from build123d import *

# Parameters (mm, degrees)
EXTRUDE1_DEPTH          = 0.25
FILLET1_R               = 0.25
CUT_EXTRUDE1_DEPTH      = 31.234789562
CUT_EXTRUDE1_DEPTH_BACK = 31.234789562
SKETCH3_W               = 12
SKETCH3_H               = 2.8


with BuildPart() as part:
    # Sketch1 → Revolve1 (revolve)
    with BuildSketch(Plane(origin=(0, 0, 0), x_dir=(0, 0, -1), z_dir=(1, 0, 0)), mode=Mode.PRIVATE) as revolve1_sk:
        with BuildLine():
            Line((0, 1.45), (2.15, 1.45))
            Line((2.15, 1.45), (2.15, 1.599999975))
            Line((2.15, 1.599999975), (3.15, 1.599999975))
            Line((3.15, 1.599999975), (3.15, 0))
            Line((3.15, 0), (-1.45, 0))
            ThreePointArc((-1.45, 0), (-1.025304833, 1.025304833), (0, 1.45))
        make_face()
    revolve(revolve1_sk.sketch.rotate(Axis((0, 0, 0), (0, 0, -1)), 90), axis=Axis((0, 0, 0), (0, 0, -1)))

    # Sketch2 → Extrude1 (add, symmetric)
    with BuildSketch(Plane(origin=(0, 0, 0), x_dir=(0, 0, -1), z_dir=(1, 0, 0))):
        with BuildLine():
            Line((3.15, 1.026953873), (3.95, 1.4))
            Line((3.95, 1.4), (6.15, 1.4))
            Line((6.15, 1.4), (6.15, 1.5))
            Line((6.15, 1.5), (7.15, 1.5))
            Line((7.15, 1.5), (7.15, 1.4))
            Line((7.15, 1.4), (30.15, 1.4))
            Line((30.15, 1.4), (30.15, 0.9))
            Line((30.15, 0.9), (7.15, 0.9))
            Line((7.15, 0.9), (7.15, 0.8))
            Line((7.15, 0.8), (6.15, 0.8))
            Line((6.15, 0.8), (6.15, 0.9))
            Line((6.15, 0.9), (4.05, 0.9))
            ThreePointArc((4.05, 0.9), (3.979289322, 0.870710678), (3.95, 0.8))
            Line((3.95, 0.8), (3.95, 0.5))
            Line((3.95, 0.5), (3.15, 0.5))
            Line((3.15, 0.5), (3.15, 1.026953873))
        make_face()
        with BuildLine():
            Line((3.95, -0.8), (3.95, -0.5))
            Line((3.95, -0.5), (3.15, -0.5))
            Line((3.15, -0.5), (3.15, -1.026953873))
            Line((3.15, -1.026953873), (3.95, -1.4))
            Line((3.95, -1.4), (6.15, -1.4))
            Line((6.15, -1.4), (6.15, -1.5))
            Line((6.15, -1.5), (7.15, -1.5))
            Line((7.15, -1.5), (7.15, -1.4))
            Line((7.15, -1.4), (30.15, -1.4))
            Line((30.15, -1.4), (30.15, -0.9))
            Line((30.15, -0.9), (7.15, -0.9))
            Line((7.15, -0.9), (7.15, -0.8))
            Line((7.15, -0.8), (6.15, -0.8))
            Line((6.15, -0.8), (6.15, -0.9))
            Line((6.15, -0.9), (4.05, -0.9))
            ThreePointArc((4.05, -0.9), (3.979289322, -0.870710678), (3.95, -0.8))
        make_face()
    extrude(amount=EXTRUDE1_DEPTH, both=True)

    # Fillet1
    fillet1_edges = [part.edges().sort_by_distance(p)[0] for p in [
        (-0.25, 0.763476937, -3.15),
        (0, 1.026953873, -3.15),
        (0, 0.5, -3.15),
        (0.25, 0.763476937, -3.15),
        (-0.25, -0.763476937, -3.15),
        (0, -0.5, -3.15),
        (0, -1.026953873, -3.15),
        (0.25, -0.763476937, -3.15),
    ]]
    fillet(fillet1_edges, radius=FILLET1_R)

    # Sketch3 → Cut-Extrude1 (cut, two sides: drawn at the far end of the back side and taken through both)
    with BuildSketch(Plane(origin=(0, 0, 0), x_dir=(0, 0, -1), z_dir=(1, 0, 0)).offset(-CUT_EXTRUDE1_DEPTH_BACK)):
        with Locations((24.15, 0)):
            Rectangle(SKETCH3_W, SKETCH3_H)
    extrude(amount=CUT_EXTRUDE1_DEPTH + CUT_EXTRUDE1_DEPTH_BACK, mode=Mode.SUBTRACT)


solid = part.part
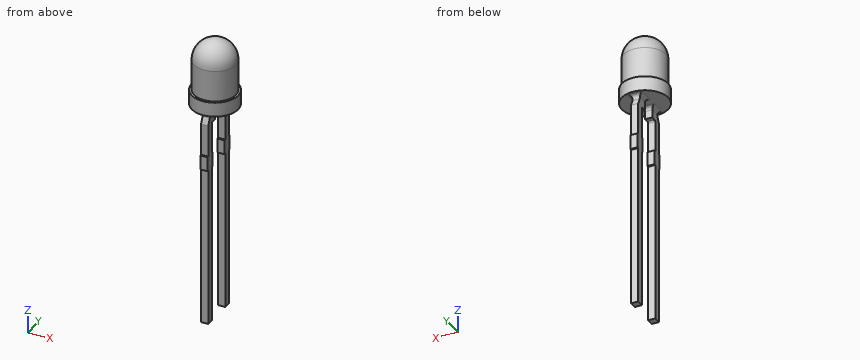
Here's how the part is built. I have some questions about the finished solid (model axes, mm). Give positions to 0.01 mm unless a question says otherwise; leave off trailing zeros. Order: outer loops, then holes, each group sorted by start corner. A loop starts at its lowest first (then second) coordinate and runs counter-clockwise, first axis right, second up. Notation, with made-up numbers: (6, 76.25) -> (18, 76.25) arc R23 cw to (18, 97.25) -> close; hole circle Ø7 at (76.25, 72.5). An arc over 180 degrees is marked (long way). Use a Markdown table: item, result. Add a question column.
Item 1: Imagine slicing it at C-C on x = -0.95. Please give me the cut outline in (y, z), plus the area to 3 significant figures.
Item 2: Imagine slicing it at B-B on y = 0. Please give me the cut outline in (x, z), plus the area to 3 significant figures.
Item 3: Will these pins go through, and if not, where does the flat tip stop? pin 1 (0.6 mm diameter, centred on x = 0, z = -7, fed in from -Y); pin 2 (1.1 mm diameter, centred on y = -1, z = -10, fed in from -X); pin 3 (0.6 mm diameter, centred on x = 0, z = -11, fed in from -Y).
Item 4: I need wall thicknesses on line 1 (X direction, y = 0.95, z = -3.75); line 2 (Y direction, x = -0.2, z = -8.25); line 3 (Y direction, x = -0.2, z = -3.25). Which ranges of each line are inside material? Lowest first, please.
Item 5: Imagine slicing it at A-A on z = -8.75. Please give me the cut outline in (x, y).
Data:
| question | item | result |
|---|---|---|
| 1 | outline | (-1.29, -3.15) -> (1.29, -3.15) -> (1.29, -2.15) -> (1.1, -2.15) -> (1.1, 0) arc R1.1 ccw to (-1.1, 0) -> (-1.1, -2.15) -> (-1.29, -2.15) -> close |
| 1 | area | 9.17 mm² |
| 2 | outline | (-1.6, -3.15) -> (1.6, -3.15) -> (1.6, -2.15) -> (1.45, -2.15) -> (1.45, 0) arc R1.45 ccw to (-1.45, 0) -> (-1.45, -2.15) -> (-1.6, -2.15) -> close |
| 2 | area | 12.7 mm² |
| 3 | pin 1 | stops at y = -1.5 |
| 3 | pin 2 | stops at x = -0.25 |
| 3 | pin 3 | stops at y = -1.4 |
| 4 | line 1 | x = -0.25 to 0.25 |
| 4 | line 2 | y = -1.4 to -0.9, 0.9 to 1.4 |
| 4 | line 3 | y = -1.22 to -0.45, 0.45 to 1.22 |
| 5 | outline | (-0.25, -1.4) -> (0.25, -1.4) -> (0.25, -0.9) -> (-0.25, -0.9) -> close; (-0.25, 0.9) -> (0.25, 0.9) -> (0.25, 1.4) -> (-0.25, 1.4) -> close |
